Read the model definition and answer for the solid it produces. Units are mm, in the model's axes. Coordinates: 2 decimals unless noted, no trailing zeros. Write each loop counter-clockwise with the first axis right and the second up, starting at its lowest first coordinate (ties: lowest second). Pieces come first, ordered by that corner, then holes. Notation, with made-up numbers: (11.25, 77) -> (52.25, 77) arc R34 ccw to (52.25, 115) -> close; hole circle Ø9 at (-38.5, 16). An arc over 180 degrees is marked (long way). Return JSON: item names as keys, results as strings.
from build123d import *

# Parameters (mm, degrees)
DODANIE_WYCI_GNI_CIE1_DEPTH = 420
WYTNIJ_WYCI_GNI_CIE1_REACH  = 427.323


with BuildPart() as part:
    # Szkic1 → Dodanie-wyciągnięcie1 (new body)
    with BuildSketch(Plane.XY):
        with BuildLine():
            Line((-12, -60), (12, -60))
            ThreePointArc((12, -60), (14.121320344, -59.121320344), (15, -57))
            Line((15, -57), (15, -3))
            ThreePointArc((15, -3), (14.121320344, -0.878679656), (12, 0))
            Line((12, 0), (-12, 0))
            ThreePointArc((-12, 0), (-14.121320344, -0.878679656), (-15, -3))
            Line((-15, -3), (-15, -57))
            ThreePointArc((-15, -57), (-14.121320344, -59.121320344), (-12, -60))
        make_face()
        with BuildLine():
            Line((-11, -3), (11, -3))
            ThreePointArc((11, -3), (11.707106781, -3.292893219), (12, -4))
            Line((12, -4), (12, -56))
            ThreePointArc((12, -56), (11.707106781, -56.707106781), (11, -57))
            Line((11, -57), (-11, -57))
            ThreePointArc((-11, -57), (-11.707106781, -56.707106781), (-12, -56))
            Line((-12, -56), (-12, -4))
            ThreePointArc((-12, -4), (-11.707106781, -3.292893219), (-11, -3))
        make_face(mode=Mode.SUBTRACT)
    extrude(amount=-DODANIE_WYCI_GNI_CIE1_DEPTH)

    # Wytnij-wyciągnięcie1: up to this face of the body (flat: up to its plane)
    wytnij_wyci_gni_cie1_end = Plane(part.part.faces().sort_by_distance((-15, -30, -210))[0])
    # Szkic2 → Wytnij-wyciągnięcie1 (cut, up to the picked face)
    with BuildSketch(Plane(origin=(15, 0, 0), x_dir=(0, 0, -1), z_dir=(1, 0, 0)), mode=Mode.PRIVATE) as wytnij_wyci_gni_cie1_sk1:
        Polygon((0, -60), (34.641016151, -60), (0, 0), align=None)
    wytnij_wyci_gni_cie1_tool1 = split(extrude(wytnij_wyci_gni_cie1_sk1.sketch, amount=-WYTNIJ_WYCI_GNI_CIE1_REACH, mode=Mode.PRIVATE), bisect_by=wytnij_wyci_gni_cie1_end, keep=Keep.BOTH, mode=Mode.PRIVATE)
    # Szkic2 → Wytnij-wyciągnięcie1 (cut, up to the picked face)
    with BuildSketch(Plane(origin=(15, 0, 0), x_dir=(0, 0, -1), z_dir=(1, 0, 0)), mode=Mode.PRIVATE) as wytnij_wyci_gni_cie1_sk2:
        Polygon((420, -60), (420, 0), (385.358983849, -60), align=None)
    wytnij_wyci_gni_cie1_tool2 = split(extrude(wytnij_wyci_gni_cie1_sk2.sketch, amount=-WYTNIJ_WYCI_GNI_CIE1_REACH, mode=Mode.PRIVATE), bisect_by=wytnij_wyci_gni_cie1_end, keep=Keep.BOTH, mode=Mode.PRIVATE)
    add(wytnij_wyci_gni_cie1_tool1.solids().sort_by(Axis((15, -40, -11.547005), (-1, 0, 0)))[0], mode=Mode.SUBTRACT)
    add(wytnij_wyci_gni_cie1_tool2.solids().sort_by(Axis((15, -40, -408.452995), (-1, 0, 0)))[0], mode=Mode.SUBTRACT)


solid = part.part
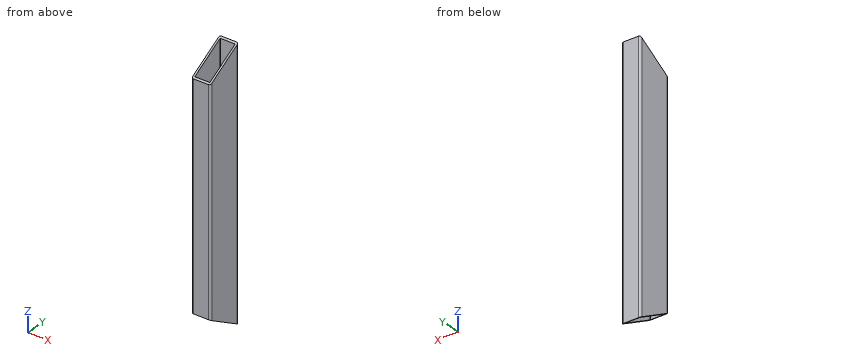
1. The part is cut by section C-C (x = -2). Determine the outline of the cut face in (y, z), then the cut area to 3 significant figures.
Taken from the geometry:
{"outline": "(-60, -385.36) -> (-57, -387.09) -> (-57, -32.91) -> (-60, -34.64) -> close; (-3, -418.27) -> (0, -420) -> (0, 0) -> (-3, -1.73) -> close", "area": "2,310 mm2"}
2. The part is cut by section A-A (z = -146.5). Determine the outline of the cut face in (x, y).
Taken from the geometry:
{"outline": "(-15, -57) arc R3 ccw to (-12, -60) -> (12, -60) arc R3 ccw to (15, -57) -> (15, -3) arc R3 ccw to (12, 0) -> (-12, 0) arc R3 ccw to (-15, -3) -> close; hole (-12, -56) arc R1 ccw to (-11, -57) -> (11, -57) arc R1 ccw to (12, -56) -> (12, -4) arc R1 ccw to (11, -3) -> (-11, -3) arc R1 ccw to (-12, -4) -> close"}
3. Consider L1, parallel to X at y = -6.5, z = -118.5; L2, parallel to Y at x = -1, z = -82; L3, parallel to Y at x = 11.5, z = -112.5. Determine where each line is inside the solid, lowest interval first.
Taken from the geometry:
{"L1": "x = -15 to -12, 12 to 15", "L2": "y = -60 to -57, -3 to 0", "L3": "y = -60 to -56.87, -3.13 to 0"}
4. The part is cut by section B-B (y = -21.5). Determine the outline of the cut face in (x, z), then the cut area to 3 significant figures.
Taken from the geometry:
{"outline": "(-15, -407.59) -> (-12, -407.59) -> (-12, -12.41) -> (-15, -12.41) -> close; (12, -407.59) -> (15, -407.59) -> (15, -12.41) -> (12, -12.41) -> close", "area": "2,370 mm2"}
5. A flat-ended cylindrical pin translates along its axis: pin 1 Ø12 at (x, y) = (-0.5, -13) entering from -Z. Find the tip coordinate at first contact, or state that the pin passes through.
Taken from the geometry:
{"pin 1": "passes through"}
